Verification items for the finished model (mm, model axes). A direction names the side the tool comes from. Give positions to 0.01 mm unless a question says otherwise; leave off trailing zeros. Write each loop counter-clockwise with the first axis right and the second up, starting at its lowest first coordinate (ties: lowest second). Pieces come first, ordered by that corner, then holes. Notation, with made-up numbers: (40.25, 20.5) - (55.25, 20.5) arc R15 ccw to (55.25, 35.5) - close; hole circle Ø11 at (78.5, 30.25). An arc over 180 degrees is marked (long way). Answer as a JSON object with one key per item and string values. Group by question number.
Item 1: Draft check along Z on faces 5 (the face through (0, 13, 5)), 6 (the face through (21, -2, 42)), 7 (the face through (-0.43, 12.15, 84.16)). Enter one of: +Z half, -Z half, draft (parallel to the pull), parting line (faces both ways), or undercut.
Item 2: Scan lines: line 1 along Z through (x, y) = (16, 11); line 2 along X through (y, z) = (13, 12.5); line 3 along X through (y, z) = (11, 72). Record each from-to range of solid material in increasing order. Write a range as [from, to].
Item 3: Sectioned sample at B-B, the plane z = 61.5. Record the boundary of the cut face in (x, y) (3 decimals).
Item 4: Go/stop test with flat-tipped pins: pin 1 (6 mm diameter, centred on x = 2.5, z = 25.5, fed in from +Y); pin 2 (16.5 mm diameter, centred on y = -1.5, z = 27.5, fed in from -X); pin 3 (12 mm diameter, centred on x = -2.5, y = -2.5, fed in from -Z); pin 4 (13 mm diameter, centred on x = 0, y = 0, fed in from -Z). Record where each tip stops, or that it passes through.
Item 5: Sectioned sample at A-A, the plane y = 0. Record the boundary of the cut face in (x, z).
Item 6: Tool access check on faces 1 (the face through (-15.91, 13.8, 74.6)), 2 (the face through (-6.977, -9.67, 41.905)), 3 (the face through (-21, -2, 42)), 4 (the face through (-3, 12, 81)). Record the directions out of +Z, -Z, +X, -X, +Y, -Y that give a thin tool (end or side, any length) a straight path to the whole face; none if there is none.
```python
from build123d import *

# Parameters (mm, degrees)
BOSS_EXTRUDE1_DEPTH         = 85
CHAMFER2_SIZE               = 1
CHAMFER3_SIZE               = 1
M5_TAPPED_HOLE1_D           = 4.2
M5_TAPPED_HOLE1_DEPTH       = 12
M5_TAPPED_HOLE1_CSINK_D     = 5.05
M5_TAPPED_HOLE1_CSINK_ANGLE = 120
M5_TAPPED_HOLE1_TIP         = 1.2618073
SKETCH6_R                   = 12
CUT_EXTRUDE1_DEPTH          = 4
SKETCH7_R                   = 12
CUT_EXTRUDE2_DEPTH          = 4
CHAMFER5_SIZE               = 1
SKETCH12_R                  = 13
CUT_EXTRUDE7_DEPTH          = 1.5
SKETCH13_R                  = 13
CUT_EXTRUDE8_DEPTH          = 1.5


with BuildPart() as part:
    # Sketch1 → Boss-Extrude1 (new body)
    with BuildSketch(Plane.XY):
        with BuildLine():
            Line((10, 19), (-10, 19))
            Line((-10, 19), (-11, 20))
            Line((-11, 20), (-22.5, 20))
            Line((-22.5, 20), (-22.5, 10))
            Line((-22.5, 10), (-21, 8.5))
            Line((-21, 8.5), (-21, -13))
            Line((-21, -13), (-8.9, -13))
            Line((-8.9, -13), (-4.999998479, -6.244999216))
            ThreePointArc((-4.999998479, -6.244999216), (0, 8), (4.999998479, -6.244999216))
            Line((4.999998479, -6.244999216), (8.9, -13))
            Line((8.9, -13), (21, -13))
            Line((21, -13), (21, 8.5))
            Line((21, 8.5), (22.5, 10))
            Line((22.5, 10), (22.5, 20))
            Line((22.5, 20), (11, 20))
            Line((11, 20), (10, 19))
        make_face()
    extrude(amount=BOSS_EXTRUDE1_DEPTH)

    # Chamfer2
    chamfer2_edges = [part.edges().sort_by_distance(p)[0] for p in [
        (-22.5, 20, 42.5),
    ]]
    chamfer(chamfer2_edges, length=CHAMFER2_SIZE)

    # Chamfer3
    chamfer3_edges = [part.edges().sort_by_distance(p)[0] for p in [
        (-21, -13, 42.5),
        (22.5, 20, 42.5),
        (21, -13, 42.5),
    ]]
    chamfer(chamfer3_edges, length=CHAMFER3_SIZE)

    # M5 Tapped Hole1
    with Locations(Plane(origin=(-16, 20, 12.5), x_dir=(0, 0, 1), z_dir=(0, 1, 0))):
        with Locations((0, 0), (0, 32), (60, 0), (60, 32)):
            CounterSinkHole(M5_TAPPED_HOLE1_D / 2, M5_TAPPED_HOLE1_CSINK_D / 2, depth=M5_TAPPED_HOLE1_DEPTH, counter_sink_angle=M5_TAPPED_HOLE1_CSINK_ANGLE)
            with Locations((0, 0, -(M5_TAPPED_HOLE1_DEPTH + M5_TAPPED_HOLE1_TIP / 2))):  # 118° drill point
                Cone(0, M5_TAPPED_HOLE1_D / 2, M5_TAPPED_HOLE1_TIP, mode=Mode.SUBTRACT)

    # Sketch6 → Cut-Extrude1 (cut)
    with BuildSketch(Plane.XY.offset(85)):
        Circle(SKETCH6_R)
    extrude(amount=-CUT_EXTRUDE1_DEPTH, mode=Mode.SUBTRACT)

    # Sketch7 → Cut-Extrude2 (cut)
    with BuildSketch(Plane(origin=(0, 0, 0), x_dir=(-1, 0, 0), z_dir=(0, 0, -1))):
        Circle(SKETCH7_R)
    extrude(amount=-CUT_EXTRUDE2_DEPTH, mode=Mode.SUBTRACT)

    # Chamfer5
    chamfer5_edges = [part.edges().sort_by_distance(p)[0] for p in [
        (0, 12, 0),
        (0, 12, 85),
    ]]
    chamfer(chamfer5_edges, length=CHAMFER5_SIZE)

    # Sketch12 → Cut-Extrude7 (cut)
    with BuildSketch(Plane.XY.offset(81)):
        Circle(SKETCH12_R)
    extrude(amount=-CUT_EXTRUDE7_DEPTH, mode=Mode.SUBTRACT)

    # Sketch13 → Cut-Extrude8 (cut)
    with BuildSketch(Plane(origin=(0, 0, 4), x_dir=(-1, 0, 0), z_dir=(0, 0, -1))):
        Circle(SKETCH13_R)
    extrude(amount=-CUT_EXTRUDE8_DEPTH, mode=Mode.SUBTRACT)


solid = part.part
```
Geometry check:
{
 "1": {"face 5": "undercut", "face 6": "draft", "face 7": "+Z half"},
 "2": {"line 1": "[0, 10.4], [14.6, 70.4], [74.6, 85]", "line 2": "[-22.5, -18.1], [-13.9, 13.9], [18.1, 22.5]", "line 3": "[-22.5, -18.04], [-13.96, 13.96], [18.04, 22.5]"},
 "3": {"outline": "(-22.5, 10) - (-21, 8.5) - (-21, -12) - (-20, -13) - (-8.9, -13) - (-5, -6.245) arc R8 cw (long way) to (5, -6.245) - (8.9, -13) - (20, -13) - (21, -12) - (21, 8.5) - (22.5, 10) - (22.5, 19) - (21.5, 20) - (11, 20) - (10, 19) - (-10, 19) - (-11, 20) - (-21.5, 20) - (-22.5, 19) - close"},
 "4": {"pin 1": "y = 19", "pin 2": "x = -21", "pin 3": "z = 5.5", "pin 4": "through"},
 "5": {"outline": "(-21, 0) - (-13, 0) - (-12, 1) - (-12, 4) - (-13, 4) - (-13, 5.5) - (-8, 5.5) - (-8, 79.5) - (-13, 79.5) - (-13, 81) - (-12, 81) - (-12, 84) - (-13, 85) - (-21, 85) - close; (8, 5.5) - (13, 5.5) - (13, 4) - (12, 4) - (12, 1) - (13, 0) - (21, 0) - (21, 85) - (13, 85) - (12, 84) - (12, 81) - (13, 81) - (13, 79.5) - (8, 79.5) - close"},
 "6": {"face 1": "+Y", "face 2": "+Z, -Z, -Y", "face 3": "+Z, -Z, -X, -Y", "face 4": "none"}
}
